For this review, take the finished solid that the model builds, in its own axes (mm). A direction names the side the tool comes from. Coordinates: 2 decimals unless noted, no trailing zeros. Loops run counter-clockwise (first coordinate to the right, second up) from the corner with the lowest first, then second, coordinate; pieces in that order, holes last. Notation, with made-up numbers: (41.25, 51) -> (45.25, 51) arc R32 cw to (45.25, 90) -> close; hole circle Ø9 at (14, 40). An arc over 180 degrees is marked (long way). One line per item, written item: value.
from build123d import *

# Parameters (mm, degrees)
CROQUIS1_R              = 1.6
SALIENTE_EXTRUIR1_DEPTH = 1.5
CROQUIS1_3_R            = 4
CROQUIS1_3_R_2          = 1.6
SALIENTE_EXTRUIR2_DEPTH = 4
CROQUIS2_R              = 1.6
CROQUIS2_W              = 115
CROQUIS2_H              = 66
SALIENTE_EXTRUIR7_DEPTH = 1.5
CORTAR_EXTRUIR1_DEPTH   = 10
REDONDEO1_R             = 1
REDONDEO2_R             = 4


with BuildPart() as part:
    # Croquis1 → Saliente-Extruir1 (new body)
    with BuildSketch(Plane(origin=(0, 0, 0), x_dir=(1, 0, 0), z_dir=(0, 1, 0))):
        with BuildLine():
            ThreePointArc((2.042155055, 3.439418953), (-3.439418964, 2.042155036), (-2.042155017, -3.439418975))
            Line((-2.042155017, -3.439418975), (79.237844983, -51.699418975))
            ThreePointArc((79.237844983, -51.699418975), (83.212910775, -51.76197886), (85.278615677, -48.365226728))
            Line((85.278615677, -48.365226728), (86.548615677, -0.105226728))
            ThreePointArc((86.548615677, -0.105226728), (85.415388884, 2.790975912), (82.55, 4))
            Line((82.55, 4), (1.098018554, 4))
            Line((1.098018554, 4), (2.042155055, 3.439418953))
        make_face()
        Polygon((77.460711282, -41.340348807), (14.571702765, -4), (78.44335204, -4), align=None, mode=Mode.SUBTRACT)
        Circle(CROQUIS1_R, mode=Mode.SUBTRACT)
        with Locations((82.55, 0)):
            Circle(CROQUIS1_R, mode=Mode.SUBTRACT)
        with Locations((81.28, -48.26)):
            Circle(CROQUIS1_R, mode=Mode.SUBTRACT)
    extrude(amount=SALIENTE_EXTRUIR1_DEPTH)

    # Croquis1<3> → Saliente-Extruir2 (add)
    with BuildSketch(Plane(origin=(0, 0, 0), x_dir=(1, 0, 0), z_dir=(0, 1, 0))):
        Circle(CROQUIS1_3_R)
        Circle(CROQUIS1_3_R_2, mode=Mode.SUBTRACT)
        with Locations((82.55, 0)):
            Circle(CROQUIS1_3_R)
        with Locations((82.55, 0)):
            Circle(CROQUIS1_3_R_2, mode=Mode.SUBTRACT)
        with Locations((81.28, -48.26)):
            Circle(CROQUIS1_3_R)
        with Locations((81.28, -48.26)):
            Circle(CROQUIS1_3_R_2, mode=Mode.SUBTRACT)
    extrude(amount=SALIENTE_EXTRUIR2_DEPTH)

    # Croquis2 → Saliente-Extruir7 (add)
    with BuildSketch(Plane.XZ):
        with BuildLine():
            Line((86.548615677, 0.105226728), (85.278615677, 48.365226728))
            ThreePointArc((85.278615677, 48.365226728), (83.212910775, 51.76197886), (79.237844983, 51.699418975))
            Line((79.237844983, 51.699418975), (-2.042155017, 3.439418975))
            ThreePointArc((-2.042155017, 3.439418975), (-3.439418975, -2.042155017), (2.042155017, -3.439418975))
            Line((2.042155017, -3.439418975), (1.098018554, -4))
            Line((1.098018554, -4), (82.55, -4))
            ThreePointArc((82.55, -4), (85.415388884, -2.790975912), (86.548615677, 0.105226728))
        make_face()
        with Locations((81.28, 48.26)):
            Circle(CROQUIS2_R, mode=Mode.SUBTRACT)
        Circle(CROQUIS2_R, mode=Mode.SUBTRACT)
        with Locations((82.55, 0)):
            Circle(CROQUIS2_R, mode=Mode.SUBTRACT)
        Polygon((14.571702765, 4), (77.460711282, 41.340348807), (78.44335204, 4), align=None, mode=Mode.SUBTRACT)
        with Locations((41.78, 19.26)):
            Rectangle(CROQUIS2_W, CROQUIS2_H)
        with BuildLine():
            ThreePointArc((85.278615677, 48.365226728), (83.212910775, 51.76197886), (79.237844983, 51.699418975))
            Line((79.237844983, 51.699418975), (-2.042155017, 3.439418975))
            ThreePointArc((-2.042155017, 3.439418975), (-3.439418975, -2.042155017), (2.042155017, -3.439418975))
            Line((2.042155017, -3.439418975), (1.098018554, -4))
            Line((1.098018554, -4), (82.55, -4))
            ThreePointArc((82.55, -4), (85.415388884, -2.790975912), (86.548615677, 0.105226728))
            Line((86.548615677, 0.105226728), (85.278615677, 48.365226728))
        make_face(mode=Mode.SUBTRACT)
    extrude(amount=-SALIENTE_EXTRUIR7_DEPTH)

    # Croquis4 → Cortar-Extruir1 (cut)
    with BuildSketch(Plane(origin=(0, 1.5, 0), x_dir=(1, 0, 0), z_dir=(0, 1, 0))):
        with BuildLine():
            Line((14.571702765, -4), (4, -4))
            Line((4, -4), (4, -49.76))
            Line((4, -49.76), (77.571900756, -49.76))
            ThreePointArc((77.571900756, -49.76), (80.51593095, -44.33365329), (85.28, -48.26))
            ThreePointArc((85.28, -48.26), (85.20634671, -49.02406905), (84.988099244, -49.76))
            Line((84.988099244, -49.76), (96.78, -49.76))
            Line((96.78, -49.76), (96.78, 5.56))
            Line((96.78, 5.56), (84.93040659, -3.214601759))
            ThreePointArc((84.93040659, -3.214601759), (83.8033142, -3.798579144), (82.55, -4))
            Line((82.55, -4), (78.44335204, -4))
            Line((78.44335204, -4), (77.460711282, -41.340348807))
            Line((77.460711282, -41.340348807), (14.571702765, -4))
        make_face()
        Polygon((91.007430697, 11.24), (-7.57, 11.24), (1.411465404, 4), (81.23022842, 4), align=None)
        Polygon((-13.22, -49.76), (-4, -49.76), (-4, -1.913370522), (-13.22, 5.518913298), align=None)
    extrude(amount=-CORTAR_EXTRUIR1_DEPTH, mode=Mode.SUBTRACT)

    # Redondeo1
    redondeo1_edges = [part.edges().sort_by_distance(p)[0] for p in [
        (4, 0.75, 4),
        (96.78, 0.75, -5.56),
        (96.78, 0.75, 49.76),
        (4, 0.75, 49.76),
        (-4, 0.75, 1.913370522),
        (-4, 0.75, 49.76),
        (-13.22, 0.75, 49.76),
        (-13.22, 0.75, -5.518913298),
        (81.23022842, 0.75, -4),
        (1.411465404, 0.75, -4),
        (-7.57, 0.75, -11.24),
        (91.007430697, 0.75, -11.24),
    ]]
    fillet(redondeo1_edges, radius=REDONDEO1_R)

    # Redondeo2
    redondeo2_edges = [part.edges().sort_by_distance(p)[0] for p in [
        (-15.72, 0.75, 52.26),
        (-15.72, 0.75, -13.74),
        (99.28, 0.75, -13.74),
        (99.28, 0.75, 52.26),
    ]]
    fillet(redondeo2_edges, radius=REDONDEO2_R)


solid = part.part
1. Take a section at C-C, the plane z = 37. Give the boundary of the cut face in (x, y).
Return value:
outline: (-15.72, 0) -> (-13.22, 0) -> (-13.22, 1.5) -> (-15.72, 1.5) -> close; (-4, 0) -> (4, 0) -> (4, 1.5) -> (-4, 1.5) -> close; (96.78, 0) -> (99.28, 0) -> (99.28, 1.5) -> (96.78, 1.5) -> close
2. For faces 1 (the flat face through (90.129, 0.76, -0.635)), 2 (the cylindrical face through (-14.517, 0.76, 51.119)), list the 3-axis set-ups (+Z, -Z, +X, -X, +Y, -Y) from which the entire face can be reached by the end or side of a thin tool; tool diameter is ignored.
Return value:
face 1: +Y, -Y
face 2: +Z, -X, +Y, -Y
3. Take a section at B-B, the plane x = 0. Give the boundary of the cut face in (y, z).
Return value:
outline: (0, -13.74) -> (1.5, -13.74) -> (1.5, -11.24) -> (0, -11.24) -> close; (0, -5.14) -> (1.5, -5.14) -> (1.5, -4) -> (4, -4) -> (4, -1.6) -> (0, -1.6) -> close; (0, 1.6) -> (4, 1.6) -> (4, 4) -> (1.5, 4) -> (1.5, 52.26) -> (0, 52.26) -> close
4. To check wall thickness, follow probe 1 along X at (y, z) = (3.1, 0); probe 2 along Z at (x, y) = (75.5, 1.1); probe 3 along X at (y, z) = (1.4, 17). State the ranges of each line that lie inside material, in increasing order. Write a range as from..to.
Return value:
probe 1: x = -4..-1.6, 1.6..4, 78.55..80.95, 84.15..86.55
probe 2: z = -13.74..-11.24, -4..4, 49.76..52.26
probe 3: x = -15.72..-13.22, -4..4, 96.78..99.28
5. Take a section at D-D, the plane x = 64. Give the boundary of the cut face in (y, z).
Return value:
outline: (0, -13.74) -> (1.5, -13.74) -> (1.5, -11.24) -> (0, -11.24) -> close; (0, -4) -> (1.5, -4) -> (1.5, 4) -> (0, 4) -> close; (0, 49.76) -> (1.5, 49.76) -> (1.5, 52.26) -> (0, 52.26) -> close
6. Take a section at A-A, the plane y = 2.85. Give the boundary of the cut face in (x, z), and give its area (3 significant figures).
Return value:
outline: circle Ø8 at (0, 0); circle Ø8 at (81.28, 48.26); circle Ø8 at (82.55, 0); hole circle Ø3.2 at (0, 0); hole circle Ø3.2 at (81.28, 48.26); hole circle Ø3.2 at (82.55, 0)
area: 127 mm2
7. The part is to be moulded in two halves that separate along Z. For faces 3 (the flat face through (-7.932, 0.76, -1.256)), 4 (the cylindrical face through (3.815, 2.732, -1.201)), 5 (the flat face through (2, 4, 0)), say which applies: pulls with the +Z half, pulls with the -Z half, needs draft (parallel to the pull), parting line crosses it, or undercut.
Return value:
face 3: undercut
face 4: parting line crosses it
face 5: needs draft
